Source: three-view drawing plus pictorial views. Frame: mm from the lowest corner of the part. A direction names the side the tool comes from. Give positions to 0.01 mm unless a question says otherwise; leave off trailing zeros. Loops run counter-clockwise (first coordinate to the right, second up) from the corner with the lowest first, then second, coordinate; pieces in that order, holes last.
1. Section C-C, the plane z = 36. Output: boundary loops of the cut face in (x, y), then the cut area to 3 significant figures.
2. Section A-A, the plane x = 24. Output: boundary loops of the cut face in (y, z).
3. Draft query along X for the marked faces 3, 4 and 5. Return one class per face: +X half, -X half, draft (parallel to the pull), parting line (faces both ways), or undercut.
4. Access query for the marked faces 1 and 2. Directions: +Z, -Z, +X, -X, +Y, -Y. A direction counts if a zero-diameter tool reaches every point of the face in a straight line with its end or side. Return the directions, or none.
5. Section B-B, the plane y = 14.25. Output: boundary loops of the cut face in (x, z).
6. Material intervals for line 1 along Z through (x, y) = (25.5, 12.25); line 2 along Z through (x, y) = (3, 5), sorted ascending.
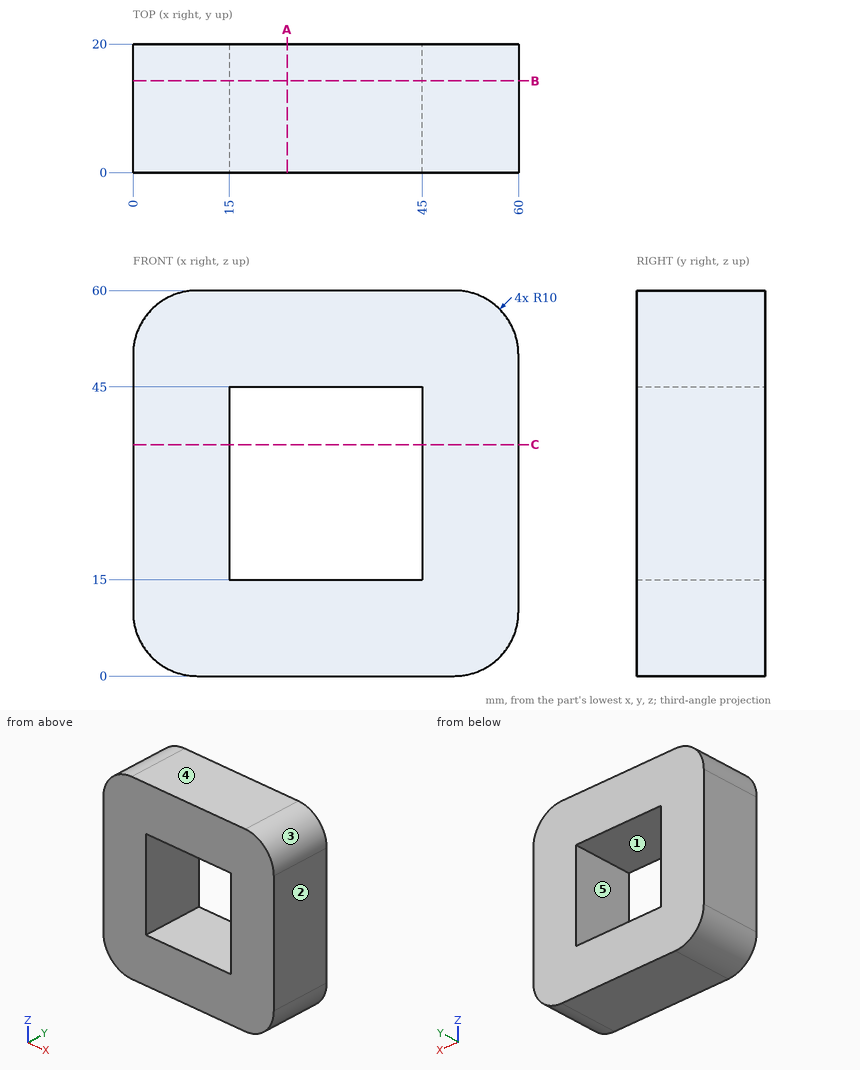
Answers below:
1. outline: (0, 0) - (15, 0) - (15, 20) - (0, 20) - close; (45, 0) - (60, 0) - (60, 20) - (45, 20) - close
1. area: 600 mm2
2. outline: (0, 0) - (20, 0) - (20, 15) - (0, 15) - close; (0, 45) - (20, 45) - (20, 60) - (0, 60) - close
3. face 3: +X half
3. face 4: draft
3. face 5: undercut
4. face 1: +Y, -Y
4. face 2: +Z, -Z, +X, +Y, -Y
5. outline: (0, 10) arc R10 ccw to (10, 0) - (50, 0) arc R10 ccw to (60, 10) - (60, 50) arc R10 ccw to (50, 60) - (10, 60) arc R10 ccw to (0, 50) - close; hole (15, 15) - (45, 15) - (45, 45) - (15, 45) - close
6. line 1: z = 0 to 15, 45 to 60
6. line 2: z = 2.86 to 57.14
